from build123d import *

# Parameters (mm, degrees)
SALIENTE_EXTRUIR5_DEPTH = 25


with BuildPart() as part:
    # Croquis1 → Saliente-Extruir5 (new body)
    with BuildSketch(Plane.XY):
        with BuildLine():
            Line((-103.421749263, -28.548605363), (-103.421749263, -38.548605363))
            Line((-103.421749263, -38.548605363), (6.578250737, -38.548605363))
            Line((6.578250737, -38.548605363), (6.578250737, -28.548605363))
            Line((6.578250737, -28.548605363), (-8.421749263, -28.548605363))
            Line((-8.421749263, -28.548605363), (-8.421749263, 41.451394637))
            Line((-8.421749263, 41.451394637), (-37.421749263, 41.451394637))
            Line((-37.421749263, 41.451394637), (-37.421749263, 56.451394637))
            Line((-37.421749263, 56.451394637), (-47.421749263, 56.451394637))
            Line((-47.421749263, 56.451394637), (-47.421749263, 32.435261406))
            ThreePointArc((-47.421749263, 32.435261406), (-26.150691812, 23.015253289), (-17.421749263, 1.451394637))
            ThreePointArc((-17.421749263, 1.451394637), (-69.985607916, -20.819662815), (-49.421749263, 32.435261406))
            Line((-49.421749263, 32.435261406), (-49.421749263, 56.380232155))
            Line((-49.421749263, 56.380232155), (-59.421749263, 56.380232155))
            Line((-59.421749263, 56.380232155), (-59.421749263, 41.704732865))
            Line((-59.421749263, 41.704732865), (-88.421749263, 41.824609442))
            Line((-88.421749263, 41.824609442), (-88.421749263, -28.548605363))
            Line((-88.421749263, -28.548605363), (-103.421749263, -28.548605363))
        make_face()
    extrude(amount=SALIENTE_EXTRUIR5_DEPTH)


solid = part.part
Could you check a few things on this model? Use its own coordinates, in mm. A direction names the side the tool comes from. Round coordinates to 2 decimals unless told otherwise and drop trailing zeros. Write each loop counter-clockwise with the first axis right and the second up, starting at its lowest first coordinate (ties: lowest second). Pieces come first, ordered by that corner, then holes. Notation, with made-up numbers: (22, 47) - (55, 47) arc R6 ccw to (55, 58) - close; hole circle Ø9 at (-19.5, 12). An arc over 180 degrees is marked (long way). Put each result on its own line as item: value. Start each with the question number.
(1) I want a section at C-C, the plane x = -56. Please give me the cut outline in (y, z), plus the area to 3 significant figures.
(2) I need wall thicknesses on probe 1 along X at (y, z) = (42.5, 14.25); probe 2 along X at (y, z) = (39.5, 13.5); probe 3 along Y at (x, z) = (-15, 13.25). Which ranges of each line are inside material? Lowest first, please.
(3) For faces 4 (the flat face through (-1, -28.549, 12)), 5 (the flat face through (-96, -28.549, 12)), 6 (the flat face through (-49, -38.549, 12)), 7 (the flat face through (-49.422, 44, 12)), which set-ups out of +Z, -Z, +X, -X, +Y, -Y let a thin tool reach every point of the face, with its end or its side?
(4) Thinking about a two-plate mould opening in X: for faces 1 (the flat face through (-42, 56.451, 12)), 2 (the flat face through (-47.422, 45, 12)), 3 (the flat face through (-8.422, 6, 12)), which applies, released by +X, released by -X, zero draft, split by the parting line, or undercut?
(5) I want a section at A-A, the plane y = -13.5. Please give me the cut outline in (x, z).
(6) I want a section at D-D, the plane x = -93. Please give me the cut outline in (y, z), plus the area to 3 significant figures.
(7) I want a section at B-B, the plane z = 3.5. Please give me the cut outline in (x, y), plus the area to 3 significant figures.
(8) Will these pins go through, and if not, where does the flat tip stop? pin 1 (12 mm diameter, centred on y = 39.5, z = 18, fed in from -X); pin 2 (7.5 mm diameter, centred on y = 49, z = 11, fed in from +X); pin 3 (7.5 mm diameter, centred on y = 12.5, z = 18.5, fed in from +X); pin 4 (1 mm diameter, centred on x = -7, y = -27.5, fed in from +Z).
Here are the results:
1. outline: (-38.55, 0) - (-28.61, 0) - (-28.61, 25) - (-38.55, 25) - close; (31.51, 0) - (56.38, 0) - (56.38, 25) - (31.51, 25) - close
1. area: 870 mm^2
2. probe 1: x = -59.42 to -49.42, -47.42 to -37.42
2. probe 2: x = -88.42 to -49.42, -47.42 to -8.42
2. probe 3: y = -38.55 to 41.45
3. face 4: +Z, -Z, +X, +Y
3. face 5: +Z, -Z, -X, +Y
3. face 6: +Z, -Z, +X, -X, -Y
3. face 7: +Z, -Z, +Y
4. face 1: zero draft
4. face 2: undercut
4. face 3: released by +X
5. outline: (-88.42, 0) - (-75.58, 0) - (-75.58, 25) - (-88.42, 25) - close; (-21.27, 0) - (-8.42, 0) - (-8.42, 25) - (-21.27, 25) - close
6. outline: (-38.55, 0) - (-28.55, 0) - (-28.55, 25) - (-38.55, 25) - close
6. area: 250 mm^2
7. outline: (-103.42, -38.55) - (6.58, -38.55) - (6.58, -28.55) - (-8.42, -28.55) - (-8.42, 41.45) - (-37.42, 41.45) - (-37.42, 56.45) - (-47.42, 56.45) - (-47.42, 32.44) arc R31 cw (long way) to (-49.42, 32.44) - (-49.42, 56.38) - (-59.42, 56.38) - (-59.42, 41.7) - (-88.42, 41.82) - (-88.42, -28.55) - (-103.42, -28.55) - close
7. area: 3,970 mm^2
8. pin 1: stops at x = -88.42
8. pin 2: stops at x = -37.42
8. pin 3: stops at x = -8.42
8. pin 4: passes through
